Here's how the part is built. I have some questions about the finished solid (model axes, mm). A direction names the side the tool comes from. Round coordinates to 2 decimals unless told otherwise and drop trailing zeros. Use one line per item in the form item = value. Start each with the question number.
1. We'd pull the mould along X, two halves only. Please class faces 1 (the cylindrical face through (115.766, -1.944, 44.175)), 2 (the flat face through (122.764, 9, 19)), 3 (the flat face through (99.491, 16, 16)): +X half, -X half, draft (parallel to the pull), parting line (faces both ways), or undercut.
2. Which directions (+Z, -Z, +X, -X, +Y, -Y) give clear straight access to the entire face, cutting with the end or side of a thin tool? Please do faces 4 (the cylindrical face through (121, 0, 35)), 5 (the cylindrical face through (-3, 0, -25)), 6 (the cylindrical face through (-17.76, 15.62, 3.47)).
3. Will these pins go through, and if not, where does the flat tip stop? pin 1 (8 mm diameter, centred on y = 30, z = 0, fed in from +X); pin 2 (10 mm diameter, centred on x = 73.5, z = -27, fed in from +Y); pin 3 (12 mm diameter, centred on y = -4.5, z = -27, fed in from +X); pin 4 (8 mm diameter, centred on x = -44, y = -20, fed in from -Z).
4. If I drill on line 1 along X through (y, z) = (-2, 22); line 2 along X through (y, z) = (-27, 25); line 3 along Y through (x, z) = (-2.75, 0), over which ranges is the centre line in solid material (lowest first)?
5. I want a section at A-A, the plane y = 0. State how many separate pieces and enclosed holes the cut face has, plus the area to 3 significant figures.
```python
from build123d import *

# Parameters (mm, degrees)
SKETCH2_R                = 3.996978994
SKETCH2_R_2              = 4.344542385
BOSS_EXTRUDE1_DEPTH      = 48
SKETCH3_R                = 2.344542385
SKETCH3_R_2              = 1.996978994
CUT_EXTRUDE1_DEPTH       = 48
SKETCH4_R                = 5
CUT_EXTRUDE2_DEPTH       = 19
CUT_EXTRUDE3_START       = 129
SKETCH4_2_R              = 5
CUT_EXTRUDE3_DEPTH       = 19
BOSS_EXTRUDE2_DEPTH      = 4
BOSS_EXTRUDE2_DEPTH_BACK = 136
SKETCH5_R                = 20
SKETCH6_R                = 16


with BuildPart() as part:
    # Sketch1 → Revolve2 (revolve)
    with BuildSketch(Plane.XY, mode=Mode.PRIVATE) as revolve2_sk:
        Polygon((99.490909091, 16), (99.490909091, 36.363636364), (13.090909091, 36.363636364), (13.090909091, 16), (-2.036363636, 16), (-2.036363636, 44.218181818), (-4.363636364, 44.218181818), (-4.363636364, 0.301244101), (-6.690909091, 0.301244101), (-6.690909091, 44.218181818), (-10.181818182, 44.218181818), (-10.181818182, 16), (-21.236363636, 16), (-21.236363636, 0), (133.818181818, 0), (133.818181818, 16), (122.763636364, 16), (122.763636364, 44.218181818), (119.272727273, 44.218181818), (119.272727273, 0.301244101), (116.945454545, 0.301244101), (116.945454545, 44.218181818), (114.618181818, 44.218181818), (114.618181818, 16), align=None)
    revolve(revolve2_sk.sketch.rotate(Axis((0, 0, 0), (-1, 0, 0)), 90), axis=Axis((0, 0, 0), (-1, 0, 0)))

    # Sketch2 → Boss-Extrude1 (add)
    with BuildSketch(Plane(origin=(0, 0, 0), x_dir=(1, 0, 0), z_dir=(0, 1, 0))):
        with Locations(Location((43.08350024, 0, 0), (0, 0, 90))):
            Circle(SKETCH2_R)
        with Locations(Location((61.504359953, 0, 0), (0, 0, 90))):
            Circle(SKETCH2_R_2)
    extrude(amount=BOSS_EXTRUDE1_DEPTH)

    # Sketch3 → Cut-Extrude1 (cut)
    with BuildSketch(Plane(origin=(0, 48, 0), x_dir=(1, 0, 0), z_dir=(0, 1, 0))):
        with Locations(Location((61.504359953, 0, 0), (0, 0, 270))):
            Circle(SKETCH3_R)
        with Locations(Location((43.08350024, 0, 0), (0, 0, 270))):
            Circle(SKETCH3_R_2)
    extrude(amount=-CUT_EXTRUDE1_DEPTH, mode=Mode.SUBTRACT)

    # Sketch4 → Cut-Extrude2 (cut)
    with BuildSketch(Plane(origin=(0, 0, 0), x_dir=(0, 0, -1), z_dir=(1, 0, 0))):
        with Locations((0, 30)):
            Circle(SKETCH4_R)
        with Locations((30, 0)):
            Circle(SKETCH4_R)
        with Locations((0, -30)):
            Circle(SKETCH4_R)
        with Locations((-30, 0)):
            Circle(SKETCH4_R)
    extrude(amount=-CUT_EXTRUDE2_DEPTH, mode=Mode.SUBTRACT)

    # Sketch4_2 → Cut-Extrude3 (cut)
    with BuildSketch(Plane(origin=(0, 0, 0), x_dir=(0, 0, -1), z_dir=(1, 0, 0)).offset(CUT_EXTRUDE3_START)):
        with Locations((0, 30)):
            Circle(SKETCH4_2_R)
        with Locations((30, 0)):
            Circle(SKETCH4_2_R)
        with Locations((0, -30)):
            Circle(SKETCH4_2_R)
        with Locations((-30, 0)):
            Circle(SKETCH4_2_R)
    extrude(amount=-CUT_EXTRUDE3_DEPTH, mode=Mode.SUBTRACT)

    # Sketch5 → Boss-Extrude2 (add, two sides: drawn at the far end of the back side and taken through both)
    with BuildSketch(Plane.ZY.offset(10.181818182).offset(-BOSS_EXTRUDE2_DEPTH_BACK)):
        with Locations(Location((0, 0, 0), (0, 0, 180))):
            Circle(SKETCH5_R)
    extrude(amount=BOSS_EXTRUDE2_DEPTH + BOSS_EXTRUDE2_DEPTH_BACK)

    # Sweep1: sweep along a path in Sketch7
    with BuildLine(Plane.XY) as sweep1_path:
        ThreePointArc((-21.236363636, 0), (-189.709160682, -49.779010206), (-274.996805421, -203.359773509))
    # Sketch6 → Sweep1 (sweep)
    with BuildSketch(Plane.ZY.offset(21.236363636)):
        Circle(SKETCH6_R)
    sweep(path=sweep1_path.line)


solid = part.part
```
Model answer:
q1.face_1 = draft
q1.face_2 = +X half
q1.face_3 = undercut
q2.face_4 = +X
q2.face_5 = -X
q2.face_6 = none
q3.pin_1 = 99.49
q3.pin_2 = 28.95
q3.pin_3 = 122.76
q3.pin_4 = through
q4.line_1 = -10.18 to -6.69, -4.36 to -2.04, 13.09 to 99.49, 114.62 to 116.95, 119.27 to 122.76
q4.line_2 = -10.18 to -6.69, -4.36 to -2.04, 114.62 to 116.95, 119.27 to 122.76
q4.line_3 = -44.22 to -35, -25 to 25, 35 to 44.22
q5.separate_pieces = 9
q5.enclosed_holes = 0
q5.area = 12,500 mm2
